Check sheet for the modelled part. Datum: model origin and axes. Units: mm. A direction names the side the tool comes from. Round coordinates to 2 decimals unless told otherwise and drop trailing zeros. Order: outer loops, then holes, each group sorted by start corner. A loop starts at its lowest first (then second) coordinate and runs counter-clockwise, first axis right, second up.
Q1. Mould release check, pull along Z, two halves, no side actions. Record for faces 3 (the cylindrical face through (2.192, 4.214, 30.915)), 4 (the cylindrical face through (5.96, -1.88, 16.51)), 5 (the flat face through (3, 4, 39.4)): +Z half, -Z half, draft (parallel to the pull), parting line (faces both ways), or undercut.
Q2. Cross-section at A-A on z = 27. Record the cut outline in (x, y), then the cut area to 3 significant figures.
Q3. Scan lines: probe 1 along Y at (x, z) = (0, 27.5); probe 2 along Y at (x, z) = (0, 29); probe 3 along X at (y, z) = (-0.75, 18.5). Record each from-to range of solid material in increasing order.
Q4. Depth check by flat-ended pin: P1, Ø2, axis at y = 0, z = 24.5, coming from the +X side; P2, Ø6, axis at x = 0.5, y = 0, coming from the +Z side; P3, Ø1, axis at y = 4.5, z = 19, coming from the -X side; P4, Ø2, axis at x = 1, z = 8.5, coming from the -Y side. Enter the tip coordinate at first touch or a pass-through.
Q5. Set-up check for faces 1 (the cylindrical face through (2.192, 4.214, 8.515)), 2 (the cylindrical face through (5.96, -1.88, 35.71)): record each of +Z, -Z, +X, -X, +Y, -Y from which the full face is reachable in a straight line by a thin tool's end or side.
Q6. Cross-section at B-B on y = -5.25. Give the number of separate pieces and of enclosed holes in the cut face, then the cut area to 3 significant figures.
from build123d import *

# Parameters (mm, degrees)
F2_R     = 4.5
F3_DEPTH = 39.4


with BuildPart() as f1:
    # F0 (on Front) → F1 (revolve)
    with BuildSketch(Plane.XZ):
        Polygon((0, 0), (6.25, 0), (6.25, 1), (4.75, 1), (4.75, 3.2), (6.25, 3.2), (6.25, 4.2), (4.75, 4.2), (4.75, 6.4), (6.25, 6.4), (6.25, 7.4), (4.75, 7.4), (4.75, 9.6), (6.25, 9.6), (6.25, 10.6), (4.75, 10.6), (4.75, 12.8), (6.25, 12.8), (6.25, 13.8), (4.75, 13.8), (4.75, 16), (6.25, 16), (6.25, 17), (4.75, 17), (4.75, 19.2), (6.25, 19.2), (6.25, 20.2), (4.75, 20.2), (4.75, 22.4), (6.25, 22.4), (6.25, 23.4), (4.75, 23.4), (4.75, 25.6), (6.25, 25.6), (6.25, 26.6), (4.75, 26.6), (4.75, 28.8), (6.25, 28.8), (6.25, 29.8), (4.75, 29.8), (4.75, 32), (6.25, 32), (6.25, 33), (4.75, 33), (4.75, 35.2), (6.25, 35.2), (6.25, 36.2), (4.75, 36.2), (4.75, 38.4), (6.25, 38.4), (6.25, 39.4), (4.75, 39.4), (0, 39.4), align=None)
    revolve(axis=Axis((0, 0, 19.7), (0, 0, -1)))

    # F2 (on face) → F3 (cut, through all)
    with BuildSketch(Plane.XY.offset(39.4)):
        Circle(F2_R)
    extrude(amount=-F3_DEPTH, mode=Mode.SUBTRACT)


solid = f1.part
Results found:
1. face 3: undercut
1. face 4: draft
1. face 5: +Z half
2. outline: circle Ø9.5 at (0, 0); hole circle Ø9 at (0, 0)
2. area: 7.26 mm2
3. probe 1: y = -4.75 to -4.5, 4.5 to 4.75
3. probe 2: y = -6.25 to -4.5, 4.5 to 6.25
3. probe 3: x = -4.69 to -4.44, 4.44 to 4.69
4. P1: stops at x = 4.75
4. P2: passes through
4. P3: stops at x = -4.77
4. P4: stops at y = -4.75
5. face 1: none
5. face 2: +Z, -Z
6. separate pieces: 13
6. enclosed holes: 0
6. area: 88.2 mm2
